```python
from build123d import *

# Parameters (mm, degrees)
F0_W     = 190
F0_H     = 40
F0_R     = 2.5
F1_DEPTH = 3
F2_W     = 30
F2_H     = 3
F3_DEPTH = 190


with BuildPart() as f1:
    # F0 (on Front) → F1 (new body)
    with BuildSketch(Plane.XZ):
        with Locations((-27.060809, 21.819512)):
            Rectangle(F0_W, F0_H)
        with Locations((-89.560809, 11.819512)):
            Circle(F0_R, mode=Mode.SUBTRACT)
        with Locations((35.439191, 11.819512)):
            Circle(F0_R, mode=Mode.SUBTRACT)
    extrude(amount=F1_DEPTH)

    # F2 (on face) → F3 (join, through all)
    with BuildSketch(Plane.YZ.offset(67.939191)):
        with Locations((15, 40.319512)):
            Rectangle(F2_W, F2_H)
    extrude(amount=-F3_DEPTH)


solid = f1.part
```
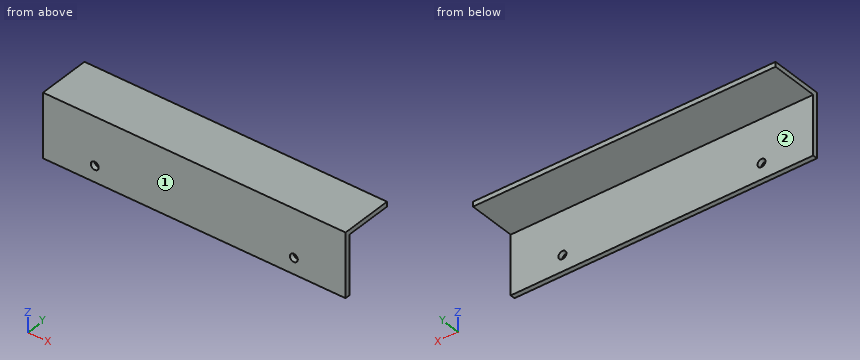
Verification items for the finished model (mm, model axes). Face numbers are marked on the shaded views. A direction names the side the tool comes from. Round coordinates to 2 decimals unless told otherwise and drop trailing zeros. Write each loop counter-clockwise with the first axis right and the second up, starting at its lowest first coordinate (ties: lowest second). Pieces come first, ordered by that corner, then holes. Notation, with made-up numbers: (82.25, 7) -> (103.25, 7) arc R17 cw to (103.25, 20) -> close; hole circle Ø2 at (48.25, 1). An arc over 180 degrees is marked (long way). Write each question's results on one line, items separated by ' | '.
Q1. Go/stop test with flat-tipped pins: pin 1 Ø15 at (x, y) = (2.5, 8) entering from -Z; pin 2 Ø8 at (x, z) = (-89.56, 11.82) entering from +Y. Record where each tip stops, or that it passes through.
Derived:
pin 1: stops at z = 38.82 | pin 2: stops at y = 0
Q2. Sectioned sample at B-B, the plane z = 30. Record the boundary of the cut face in (x, y).
Derived:
outline: (-122.06, -3) -> (67.94, -3) -> (67.94, 0) -> (-122.06, 0) -> close
Q3. Thickness scan on probe 1 along Y at (x, z) = (-80, 24); probe 2 along Z at (x, y) = (46, 5). Record the ranges inside material, lowest first.
Derived:
probe 1: y = -3 to 0 | probe 2: z = 38.82 to 41.82
Q4. Sectioned sample at C-C, the plane x = -48. Record the boundary of the cut face in (y, z), and give its area (3 significant figures).
Derived:
outline: (-3, 1.82) -> (0, 1.82) -> (0, 38.82) -> (30, 38.82) -> (30, 41.82) -> (-3, 41.82) -> close | area: 210 mm²
Q5. Access from +Z, -Z, +X, -X, +Y, -Y to the whole of each face (thin tool, end or side, straight path). Record for the marked faces 1 and 2.
Derived:
face 1: +Z, -Z, +X, -X, -Y | face 2: -Z, +X, -X, +Y
Q6. Sectioned sample at D-D, the plane y = 10. Record the boundary of the cut face in (x, z), and give its area (3 significant figures).
Derived:
outline: (-122.06, 38.82) -> (67.94, 38.82) -> (67.94, 41.82) -> (-122.06, 41.82) -> close | area: 570 mm²
Q7. Sectioned sample at A-A, the plane x = -90. Record the boundary of the cut face in (y, z).
Derived:
outline: (-3, 1.82) -> (0, 1.82) -> (0, 9.36) -> (-3, 9.36) -> close; (-3, 14.28) -> (0, 14.28) -> (0, 38.82) -> (30, 38.82) -> (30, 41.82) -> (-3, 41.82) -> close
